Design review of the part built by this model. Coordinates are the model's own, in mm. Face numbers are marked on the shaded views. A direction names the side the tool comes from. Coordinates: 2 decimals unless noted, no trailing zeros. Write each loop counter-clockwise with the first axis right and the second up, starting at its lowest first coordinate (ties: lowest second). Pieces come first, ordered by that corner, then holes. Notation, with made-up numbers: (4, 24) -> (14, 24) arc R17 cw to (14, 39) -> close; hole circle Ø4 at (-16.5, 28.25). An arc over 180 degrees is marked (long way). Answer in a Markdown table with one row per item. Add a question column.
Item 1: Draft analysis for pull direction Z (two halves, no side actions). For the marked faces 5, 6 and 7, state which applies: released by +Z, released by -Z, zero draft, split by the parting line, or undercut.
Item 2: To check wall thickness, follow line 1 (Z direction, x = -11, y = 3); line 2 (Y direction, x = -10.75, z = -1.75); line 3 (X direction, y = -0.25, z = 2.75). State the ranges of each line that lie inside material, in increasing order.
Item 3: Take a section at A-A, the plane x = -4.5. Write out the cut boundary in (y, z), and give its area (3 significant figures).
Item 4: Clearance check with flat-ended pins moving along their axes: P1, Ø6, axis at x = -3.5, z = 0, coming from the -Y side; P2, Ø0.8, axis at x = -10.5, y = 4, coming from the +Z side; P3, Ø4, axis at x = -1, z = -3, coming from the +Y side. State where each tip first meets the part, or that it passes through.
Item 5: Take a section at B-B, the plane x = 4.5. Write out the cut boundary in (y, z).
Item 6: For the marked faces 1, 2, 3 and 4, list the 3-axis set-ups (+Z, -Z, +X, -X, +Y, -Y) from which the entire face can be reached by the end or side of a thin tool; tool diameter is ignored.
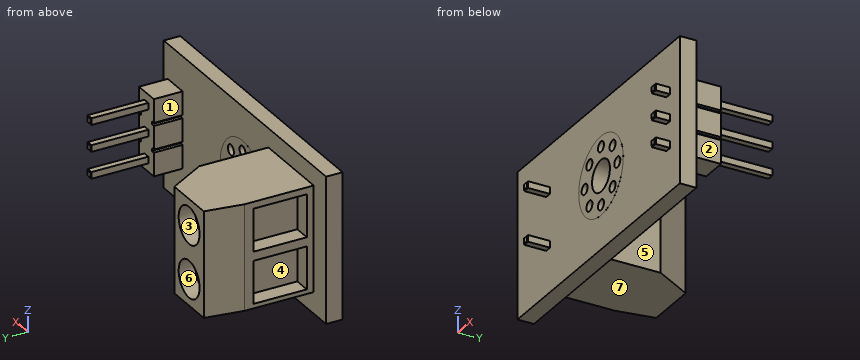
from build123d import *

# Parameters (mm, degrees)
SKETCH1_W                = 27.2923
SKETCH1_H                = 13.9192
BOSS_EXTRUDE1_DEPTH      = 0.7874
SKETCH2_R                = 1.5
SKETCH2_R_2              = 0.5
CUT_EXTRUDE1_DEPTH       = 16.399137542
SKETCH3_W                = 2.5
SKETCH3_H                = 7.3
BOSS_EXTRUDE2_DEPTH      = 2.75
SKETCH4_W                = 0.35
SKETCH4_H                = 0.29
CUT_EXTRUDE2_DEPTH       = 2.75
BOSS_EXTRUDE3_DEPTH      = 5.5
BOSS_EXTRUDE3_DEPTH_BACK = 5.7726
SKETCH5_W                = 0.635
SKETCH5_H                = 0.635
BOSS_EXTRUDE4_START      = 0.00254
SKETCH6_R                = 3.741578583
SKETCH6_R_2              = 0.5
SKETCH6_R_3              = 1.5
BOSS_EXTRUDE4_DEPTH      = 0.00254
SKETCH7_W                = 7.62
SKETCH7_H                = 10.0711
BOSS_EXTRUDE5_DEPTH      = 10.16
CUT_EXTRUDE3_DEPTH       = 19.82814406
CUT_EXTRUDE3_DEPTH_BACK  = 19.82814406
SKETCH9_R                = 1.7526
CUT_EXTRUDE4_DEPTH       = 1.6002
SKETCH10_W               = 0.635
SKETCH10_H               = 0.635
BOSS_EXTRUDE6_DEPTH      = 3.7338
CHAMFER1_SIZE            = 0.0762
SKETCH11_W               = 4.064
SKETCH11_H               = 5.08
CUT_EXTRUDE5_DEPTH       = 1.6002


with BuildPart() as part:
    # Sketch1 → Boss-Extrude1 (new, symmetric)
    with BuildSketch(Plane(origin=(0, 0, 0), x_dir=(1, 0, 0), z_dir=(0, 1, 0))):
        Rectangle(SKETCH1_W, SKETCH1_H)
    extrude(amount=BOSS_EXTRUDE1_DEPTH, both=True)

    # Sketch2 → Cut-Extrude1 (cut, through all)
    with BuildSketch(Plane(origin=(0, 0.7874, 0), x_dir=(1, 0, 0), z_dir=(0, 1, 0))):
        with Locations(Location((0.40385, 0, 0), (0, 0, 270))):
            Circle(SKETCH2_R)
        with Locations(Location((0.40385, 2.75, 0), (0, 0, 270))):
            Circle(SKETCH2_R_2)
        with Locations(Location((2.348393648, 1.944543648, 0), (0, 0, 270))):
            Circle(SKETCH2_R_2)
        with Locations(Location((3.15385, 0, 0), (0, 0, 270))):
            Circle(SKETCH2_R_2)
        with Locations(Location((2.348393648, -1.944543648, 0), (0, 0, 270))):
            Circle(SKETCH2_R_2)
        with Locations(Location((0.40385, -2.75, 0), (0, 0, 270))):
            Circle(SKETCH2_R_2)
        with Locations(Location((-1.540693648, -1.944543648, 0), (0, 0, 270))):
            Circle(SKETCH2_R_2)
        with Locations(Location((-2.34615, 0, 0), (0, 0, 270))):
            Circle(SKETCH2_R_2)
        with Locations(Location((-1.540693648, 1.944543648, 0), (0, 0, 270))):
            Circle(SKETCH2_R_2)
    extrude(amount=-CUT_EXTRUDE1_DEPTH, mode=Mode.SUBTRACT)

    # Sketch3 → Boss-Extrude2 (add)
    with BuildSketch(Plane(origin=(0, 0.7874, 0), x_dir=(1, 0, 0), z_dir=(0, 1, 0))):
        with Locations((11.71615, 0)):
            Rectangle(SKETCH3_W, SKETCH3_H)
    extrude(amount=BOSS_EXTRUDE2_DEPTH)

    # Sketch4 → Cut-Extrude2 (cut)
    with BuildSketch(Plane(origin=(0, 3.5374, 0), x_dir=(1, 0, 0), z_dir=(0, 1, 0))):
        with Locations((10.64115, 1.261418)):
            Rectangle(SKETCH4_W, SKETCH4_H)
        with Locations((10.64115, -1.261418)):
            Rectangle(SKETCH4_W, SKETCH4_H)
        with Locations((12.79115, -1.261418)):
            Rectangle(SKETCH4_W, SKETCH4_H)
        with Locations((12.79115, 1.261418)):
            Rectangle(SKETCH4_W, SKETCH4_H)
    extrude(amount=-CUT_EXTRUDE2_DEPTH, mode=Mode.SUBTRACT)

    # Sketch5 → Boss-Extrude3 (add, two sides: drawn at the far end of the back side and taken through both)
    with BuildSketch(Plane(origin=(0, 3.5374, 0), x_dir=(1, 0, 0), z_dir=(0, 1, 0)).offset(-BOSS_EXTRUDE3_DEPTH_BACK)):
        with Locations((11.71615, 0)):
            Rectangle(SKETCH5_W, SKETCH5_H)
        with Locations((11.71615, 2.54)):
            Rectangle(SKETCH5_W, SKETCH5_H)
        with Locations((11.71615, -2.54)):
            Rectangle(SKETCH5_W, SKETCH5_H)
    extrude(amount=BOSS_EXTRUDE3_DEPTH + BOSS_EXTRUDE3_DEPTH_BACK)

    # Sketch6 → Boss-Extrude4 (add)
    with BuildSketch(Plane(origin=(0, 0.7874, 0), x_dir=(1, 0, 0), z_dir=(0, 1, 0)).offset(BOSS_EXTRUDE4_START)):
        with Locations(Location((0.40385, 0, 0), (0, 0, 270))):
            Circle(SKETCH6_R)
        with Locations(Location((-2.34615, 0, 0), (0, 0, 270))):
            Circle(SKETCH6_R_2, mode=Mode.SUBTRACT)
        with Locations(Location((-1.540693648, -1.944543648, 0), (0, 0, 270))):
            Circle(SKETCH6_R_2, mode=Mode.SUBTRACT)
        with Locations(Location((0.40385, -2.75, 0), (0, 0, 270))):
            Circle(SKETCH6_R_2, mode=Mode.SUBTRACT)
        with Locations(Location((2.348393648, -1.944543648, 0), (0, 0, 270))):
            Circle(SKETCH6_R_2, mode=Mode.SUBTRACT)
        with Locations(Location((3.15385, 0, 0), (0, 0, 270))):
            Circle(SKETCH6_R_2, mode=Mode.SUBTRACT)
        with Locations(Location((2.348393648, 1.944543648, 0), (0, 0, 270))):
            Circle(SKETCH6_R_2, mode=Mode.SUBTRACT)
        with Locations(Location((0.40385, 0, 0), (0, 0, 270))):
            Circle(SKETCH6_R_3, mode=Mode.SUBTRACT)
        with Locations(Location((-1.540693648, 1.944543648, 0), (0, 0, 270))):
            Circle(SKETCH6_R_2, mode=Mode.SUBTRACT)
        with Locations(Location((0.40385, 2.75, 0), (0, 0, 270))):
            Circle(SKETCH6_R_2, mode=Mode.SUBTRACT)
    boss_extrude4 = extrude(amount=-BOSS_EXTRUDE4_DEPTH)

    # Mirror1: Boss-Extrude4 across plane
    add(boss_extrude4.mirror(Plane.ZX))

    # Sketch7 → Boss-Extrude5 (add)
    with BuildSketch(Plane(origin=(0, 0.7874, 0), x_dir=(1, 0, 0), z_dir=(0, 1, 0))):
        with Locations((-7.75335, -0.10795)):
            Rectangle(SKETCH7_W, SKETCH7_H)
    extrude(amount=BOSS_EXTRUDE5_DEPTH)

    # Sketch8 → Cut-Extrude3 (cut, two sides: drawn at the far end of the back side and taken through both)
    with BuildSketch(Plane.XY.offset(-CUT_EXTRUDE3_DEPTH_BACK)):
        Polygon((-6.01345, 10.9474), (-3.94335, 7.3914), (-3.94335, 10.9474), align=None)
        Polygon((-10.96645, 10.9474), (-11.56335, 10.9474), (-11.56335, 7.3914), align=None)
    extrude(amount=CUT_EXTRUDE3_DEPTH + CUT_EXTRUDE3_DEPTH_BACK, mode=Mode.SUBTRACT)

    # Sketch9 → Cut-Extrude4 (cut)
    with BuildSketch(Plane(origin=(0, 10.9474, 0), x_dir=(1, 0, 0), z_dir=(0, 1, 0))):
        with Locations(Location((-8.48995, 2.43205, 0), (0, 0, 270))):
            Circle(SKETCH9_R)
        with Locations(Location((-8.48995, -2.64795, 0), (0, 0, 270))):
            Circle(SKETCH9_R)
    extrude(amount=-CUT_EXTRUDE4_DEPTH, mode=Mode.SUBTRACT)

    # Sketch10 → Boss-Extrude6 (add)
    with BuildSketch(Plane(origin=(0, 0.7874, 0), x_dir=(1, 0, 0), z_dir=(0, 1, 0))):
        with Locations((-8.48995, 2.43205)):
            Rectangle(SKETCH10_W, SKETCH10_H)
        with Locations((-8.48995, -2.64795)):
            Rectangle(SKETCH10_W, SKETCH10_H)
    extrude(amount=-BOSS_EXTRUDE6_DEPTH)

    # Chamfer1
    chamfer1_edges = [part.edges().sort_by_distance(p)[0] for p in [
        (12.03365, -2.2352, 0),
        (11.71615, -2.2352, 0.3175),
        (11.39865, -2.2352, 0),
        (11.71615, -2.2352, -0.3175),
        (12.03365, 9.0374, 0),
        (11.71615, 9.0374, -0.3175),
        (11.39865, 9.0374, 0),
        (11.71615, 9.0374, 0.3175),
        (12.03365, -2.2352, -2.54),
        (11.71615, -2.2352, -2.2225),
        (11.39865, -2.2352, -2.54),
        (11.71615, -2.2352, -2.8575),
        (12.03365, 9.0374, -2.54),
        (11.71615, 9.0374, -2.8575),
        (11.39865, 9.0374, -2.54),
        (11.71615, 9.0374, -2.2225),
        (12.03365, -2.2352, 2.54),
        (11.71615, -2.2352, 2.8575),
        (11.39865, -2.2352, 2.54),
        (11.71615, -2.2352, 2.2225),
        (12.03365, 9.0374, 2.54),
        (11.71615, 9.0374, 2.2225),
        (11.39865, 9.0374, 2.54),
        (11.71615, 9.0374, 2.8575),
        (-8.17245, -2.9464, -2.43205),
        (-8.48995, -2.9464, -2.11455),
        (-8.80745, -2.9464, -2.43205),
        (-8.48995, -2.9464, -2.74955),
        (-8.17245, -2.9464, 2.64795),
        (-8.48995, -2.9464, 2.96545),
        (-8.80745, -2.9464, 2.64795),
        (-8.48995, -2.9464, 2.33045),
    ]]
    chamfer(chamfer1_edges, length=CHAMFER1_SIZE)

    # Sketch11 → Cut-Extrude5 (cut)
    with BuildSketch(Plane.ZY.offset(11.56335)):
        with Locations((-2.4638, 3.987287249)):
            Rectangle(SKETCH11_W, SKETCH11_H)
        with Locations((2.4638, 3.987287249)):
            Rectangle(SKETCH11_W, SKETCH11_H)
    extrude(amount=-CUT_EXTRUDE5_DEPTH, mode=Mode.SUBTRACT)


solid = part.part
Answers:
| question | item | result |
|---|---|---|
| 1 | face 5 | zero draft |
| 1 | face 6 | undercut |
| 1 | face 7 | released by -Z |
| 2 | line 1 | z = -4.93 to -4.5, -0.43 to 0.43, 4.5 to 5.14 |
| 2 | line 2 | y = -0.79 to 1.45, 6.53 to 10.95 |
| 2 | line 3 | x = -13.65 to -0.1, 0.9 to 13.65 |
| 3 | outline | (-0.79, -6.96) -> (0.79, -6.96) -> (0.79, -4.93) -> (8.35, -4.93) -> (8.35, 5.14) -> (0.79, 5.14) -> (0.79, 6.96) -> (-0.79, 6.96) -> close |
| 3 | area | 98.1 mm^2 |
| 4 | P1 | stops at y = -0.79 |
| 4 | P2 | stops at z = 5.14 |
| 4 | P3 | stops at y = 0.79 |
| 5 | outline | (-0.79, -6.96) -> (0.79, -6.96) -> (0.79, 6.96) -> (-0.79, 6.96) -> close |
| 6 | face 1 | +Z, -Z, +Y |
| 6 | face 2 | +Z, -Z, +X, +Y |
| 6 | face 3 | +Y |
| 6 | face 4 | -X |
